from build123d import *

# Parameters (mm, degrees)
BOSS_EXTRUDE1_DEPTH = 20
SKETCH2_R           = 6.25
CUT_EXTRUDE1_DEPTH  = 11
SKETCH2_3_R         = 2.15
CUT_EXTRUDE2_DEPTH  = 31
CUT_EXTRUDE3_START  = -15
SKETCH2_4_R         = 2.15
CUT_EXTRUDE3_DEPTH  = 15
SKETCH3_R           = 2.25
CUT_EXTRUDE4_DEPTH  = 25.919871589
SKETCH4_R           = 4
CUT_EXTRUDE5_DEPTH  = 4


with BuildPart() as part:
    # Sketch1 → Boss-Extrude1 (new body)
    with BuildSketch(Plane(origin=(0, 0, 0), x_dir=(1, 0, 0), z_dir=(0, 1, 0))):
        with BuildLine():
            ThreePointArc((-7.5, -6.614378278), (0, -10), (7.5, -6.614378278))
            ThreePointArc((7.5, -6.614378278), (10.307771776, -4.826585903), (13.636363636, -4.810456929))
            ThreePointArc((13.636363636, -4.810456929), (20, 0), (13.636363636, 4.810456929))
            ThreePointArc((13.636363636, 4.810456929), (10.307771776, 4.826585903), (7.5, 6.614378278))
            ThreePointArc((7.5, 6.614378278), (0, 10), (-7.5, 6.614378278))
            ThreePointArc((-7.5, 6.614378278), (-10.307771776, 4.826585903), (-13.636363636, 4.810456929))
            ThreePointArc((-13.636363636, 4.810456929), (-20, 0), (-13.636363636, -4.810456929))
            ThreePointArc((-13.636363636, -4.810456929), (-10.307771776, -4.826585903), (-7.5, -6.614378278))
        make_face()
    extrude(amount=BOSS_EXTRUDE1_DEPTH)

    # Sketch2 → Cut-Extrude1 (cut)
    with BuildSketch(Plane(origin=(0, 20, 0), x_dir=(1, 0, 0), z_dir=(0, 1, 0))):
        with Locations(Location((0, 0, 0), (0, 0, 270))):
            Circle(SKETCH2_R)
    extrude(amount=-CUT_EXTRUDE1_DEPTH, mode=Mode.SUBTRACT)

    # Sketch2<3> → Cut-Extrude2 (cut, through all)
    with BuildSketch(Plane(origin=(0, 20, 0), x_dir=(1, 0, 0), z_dir=(0, 1, 0))):
        with Locations(Location((-15, 0, 0), (0, 0, 270))):
            Circle(SKETCH2_3_R)
        with Locations(Location((15, 0, 0), (0, 0, 270))):
            Circle(SKETCH2_3_R)
    extrude(amount=-CUT_EXTRUDE2_DEPTH, mode=Mode.SUBTRACT)

    # Sketch2<4> → Cut-Extrude3 (cut)
    # profile 1 of 2: a face of its own
    with BuildSketch(Plane(origin=(0, 20, 0), x_dir=(1, 0, 0), z_dir=(0, 1, 0)).offset(CUT_EXTRUDE3_START)):
        with BuildLine():
            Line((-10.669872981, 0), (-12.834936491, 3.75))
            Line((-12.834936491, 3.75), (-12.727737442, 4.627302245))
            ThreePointArc((-12.727737442, 4.627302245), (-13.185592631, 4.701307351), (-13.636363636, 4.810456929))
            ThreePointArc((-13.636363636, 4.810456929), (-20, 0), (-13.636363636, -4.810456929))
            ThreePointArc((-13.636363636, -4.810456929), (-13.238538502, -4.712228262), (-12.834936491, -4.641382481))
            Line((-12.834936491, -4.641382481), (-12.834936491, -3.75))
            Line((-12.834936491, -3.75), (-10.669872981, 0))
        make_face()
        with Locations(Location((-15, 0, 0), (0, 0, 270))):
            Circle(SKETCH2_4_R, mode=Mode.SUBTRACT)
    # profile 2 of 2: a face of its own
    with BuildSketch(Plane(origin=(0, 20, 0), x_dir=(1, 0, 0), z_dir=(0, 1, 0)).offset(CUT_EXTRUDE3_START)):
        with BuildLine():
            ThreePointArc((13.636363636, 4.810456929), (13.238538502, 4.712228262), (12.834936491, 4.641382481))
            Line((12.834936491, 4.641382481), (12.834936491, 3.75))
            Line((12.834936491, 3.75), (10.669872981, 0))
            Line((10.669872981, 0), (12.834936491, -3.75))
            Line((12.834936491, -3.75), (12.727737442, -4.627302245))
            ThreePointArc((12.727737442, -4.627302245), (13.185592631, -4.701307351), (13.636363636, -4.810456929))
            ThreePointArc((13.636363636, -4.810456929), (20, 0), (13.636363636, 4.810456929))
        make_face()
        with Locations(Location((15, 0, 0), (0, 0, 270))):
            Circle(SKETCH2_4_R, mode=Mode.SUBTRACT)
    extrude(amount=CUT_EXTRUDE3_DEPTH, mode=Mode.SUBTRACT)

    # Sketch3 → Cut-Extrude4 (cut, through all)
    with BuildSketch(Plane(origin=(0, 9, 0), x_dir=(1, 0, 0), z_dir=(0, 1, 0))):
        with Locations(Location((0, 0, 0), (0, 0, 270))):
            Circle(SKETCH3_R)
    extrude(amount=-CUT_EXTRUDE4_DEPTH, mode=Mode.SUBTRACT)

    # Sketch4 → Cut-Extrude5 (cut)
    with BuildSketch(Plane.XZ):
        with Locations(Location((0, 0, 0), (0, 0, 270))):
            Circle(SKETCH4_R)
    extrude(amount=-CUT_EXTRUDE5_DEPTH, mode=Mode.SUBTRACT)


solid = part.part
Check sheet for the modelled part. Datum: model origin and axes. Units: mm. A direction names the side the tool comes from. Give positions to 0.01 mm unless a question says otherwise; leave off trailing zeros. Loops run counter-clockwise (first coordinate to the right, second up) from the corner with the lowest first, then second, coordinate; pieces in that order, holes last. Notation, with made-up numbers: M 33,86 L 70,86 A15 cw 70,97 Z; hole C 89,-15 d2. An arc over 180 degrees is marked long. Answer as a JSON object with one key per item and string values. Group by question number.
Q1. Release check for a two-part mould opening along X. For faces 1 (the cylindrical face through (1.88, 14.58, 5.96)), 2 (the flat face through (12.782, 12.395, 4.183)), 3 (the flat face through (0, 20, -7)), 4 (the flat face through (-3, 9, 0)) record: released by +X, released by -X, zero draft, split by the parting line, or undercut.
Q2. Cross-section at A-A on x = -15. Record the cut outline in (y, z), then the cut area to 3 significant figures.
Q3. Go/stop test with flat-tipped pins: P1, Ø12, axis at y = 3.5, z = -7, coming from the +X side; P2, Ø1, axis at y = 11.5, z = -4, coming from the +X side; P3, Ø8, axis at x = 11, y = 5, coming from the +Z side; P4, Ø12, axis at x = 10.5, z = 5.5, coming from the -Y side. Record where each tip stops, or that it passes through.
Q4. Cross-section at C-C on y = 15. Record the cut outline in (x, z), then the cut area to 3 significant figures.
Q5. Cross-section at D-D on x = -5. Record the cut outline in (y, z), then the cut area to 3 significant figures.
Q6. Material ranges on line 1 along X through (y, z) = (13.25, 0); line 2 along X through (y, z) = (7.1, 0); line 3 along Y through (x, z) = (15, -3), recorded low to high. Write a range as [from, to].
Q7. Cross-section at B-B on y = 7. Record the cut outline in (x, z), then the cut area to 3 significant figures.
Q8. Access from +Z, -Z, +X, -X, +Y, -Y to the whole of each face (thin tool, end or side, straight path). Record for faces 5 (the flat face through (-2, 4, -2)), 6 (the flat face through (-17.5, 5, -0.1)), 7 (the flat face through (11.74, 12.4, 1.85)), 8 (the flat face through (12.835, 12, -4)).
Evaluation:
{
 "1": {"face 1": "undercut", "face 2": "released by +X", "face 3": "zero draft", "face 4": "undercut"},
 "2": {"outline": "M 0,-5 L 5,-5 L 5,-2.15 L 0,-2.15 Z; M 0,2.15 L 5,2.15 L 5,5 L 0,5 Z", "area": "28.5 mm2"},
 "3": {"P1": "stops at x = 19.9", "P2": "stops at x = 12.83", "P3": "stops at z = 7.14", "P4": "stops at y = 0"},
 "4": {"outline": "M -12.83,-3.75 L -12.73,-4.63 A6 cw -7.5,-6.61 A10 ccw 7.5,-6.61 A6 cw 12.83,-4.64 L 12.83,-3.75 L 10.67,0 L 12.83,3.75 L 12.73,4.63 A6 cw 7.5,6.61 A10 ccw -7.5,6.61 A6 cw -12.83,4.64 L -12.83,3.75 L -10.67,0 Z; hole C 0,0 d12.5", "area": "239 mm2"},
 "5": {"outline": "M 0,-8.66 L 20,-8.66 L 20,-3.75 L 9,-3.75 L 9,3.75 L 20,3.75 L 20,8.66 L 0,8.66 Z", "area": "264 mm2"},
 "6": {"line 1": "x = [-10.67, -6.25], [6.25, 10.67]", "line 2": "x = [-10.67, -2.25], [2.25, 10.67]", "line 3": "y = [0, 5]"},
 "7": {"outline": "M -12.83,-3.75 L -12.73,-4.63 A6 cw -7.5,-6.61 A10 ccw 7.5,-6.61 A6 cw 12.83,-4.64 L 12.83,-3.75 L 10.67,0 L 12.83,3.75 L 12.73,4.63 A6 cw 7.5,6.61 A10 ccw -7.5,6.61 A6 cw -12.83,4.64 L -12.83,3.75 L -10.67,0 Z; hole C 0,0 d4.5", "area": "346 mm2"},
 "8": {"face 5": "-Y", "face 6": "-X, +Y", "face 7": "+X, +Y", "face 8": "+Z, -Z, +X, +Y"}
}
